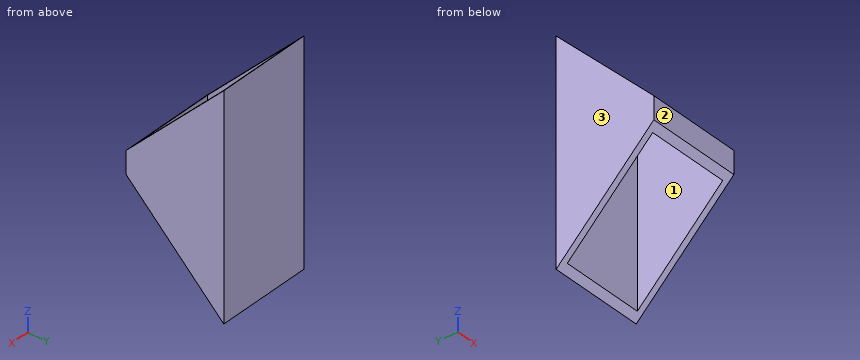
```python
from build123d import *

# Parameters (mm, degrees)
CROQUIS2_W              = 76.2
CROQUIS2_H              = 76.2
CROQUIS2_W_2            = 66.675
CROQUIS2_H_2            = 66.675
SALIENTE_EXTRUIR1_DEPTH = 170
CORTAR_EXTRUIR1_REACH   = 203.278


with BuildPart() as part:
    # Croquis2 → Saliente-Extruir1 (new body)
    with BuildSketch(Plane.XY):
        with Locations((38.1, -38.1)):
            Rectangle(CROQUIS2_W, CROQUIS2_H)
        with Locations((38.1, -38.1)):
            Rectangle(CROQUIS2_W_2, CROQUIS2_H_2, mode=Mode.SUBTRACT)
    extrude(amount=-SALIENTE_EXTRUIR1_DEPTH)

    # Cortar-Extruir1: up to this face of the body (flat: up to its plane)
    cortar_extruir1_end = Plane(part.part.faces().sort_by_distance((0, -38.1, -85))[0])
    # Croquis3 → Cortar-Extruir1 (cut, up to the picked face)
    with BuildSketch(Plane(origin=(76.2, 0, 0), x_dir=(0, 0, -1), z_dir=(1, 0, 0)), mode=Mode.PRIVATE) as cortar_extruir1_sk1:
        Polygon((0, 0), (76.2, -76.2), (0, -76.2), align=None)
    cortar_extruir1_tool1 = split(extrude(cortar_extruir1_sk1.sketch, amount=-CORTAR_EXTRUIR1_REACH, mode=Mode.PRIVATE), bisect_by=cortar_extruir1_end, keep=Keep.BOTH, mode=Mode.PRIVATE)
    # Croquis3 → Cortar-Extruir1 (cut, up to the picked face)
    with BuildSketch(Plane(origin=(76.2, 0, 0), x_dir=(0, 0, -1), z_dir=(1, 0, 0)), mode=Mode.PRIVATE) as cortar_extruir1_sk2:
        Polygon((170, 0), (93.8, -76.2), (170, -76.2), align=None)
    cortar_extruir1_tool2 = split(extrude(cortar_extruir1_sk2.sketch, amount=-CORTAR_EXTRUIR1_REACH, mode=Mode.PRIVATE), bisect_by=cortar_extruir1_end, keep=Keep.BOTH, mode=Mode.PRIVATE)
    add(cortar_extruir1_tool1.solids().sort_by(Axis((76.2, -50.8, -25.4), (-1, 0, 0)))[0], mode=Mode.SUBTRACT)
    add(cortar_extruir1_tool2.solids().sort_by(Axis((76.2, -50.8, -144.6), (-1, 0, 0)))[0], mode=Mode.SUBTRACT)


solid = part.part
```
Verification items for the finished model (mm, model axes). Face numbers are marked on the shaded views. Coordinates: 2 decimals unless noted, no trailing zeros. Loops run counter-clockwise (first coordinate to the right, second up) from the corner with the lowest first, then second, coordinate; pieces in that order, holes last. Notation, with made-up numbers: (71.5, 47) -> (124.5, 47) arc R17 ccw to (124.5, 65) -> close; hole circle Ø7 at (28, 39). An arc over 180 degrees is marked (long way). Answer in a Markdown table with one row per item. Add a question column.
1. Section check A-A, the plane y = -56. Enter the section's corners in (x, z), then the cut area to 3 significant figures.
2. Material ranges on probe 1 along X at (y, z) = (-40.5, -114.5); probe 2 along Y at (x, z) = (52, -51); probe 3 along Z at (x, y) = (71.5, -47), recorded low to high. Write a range as [from, to].
3. Depth check by flat-ended pin: P1, Ø12, axis at x = 58, z = -19.5, coming from the +Y side; P2, Ø12, axis at x = 44.5, z = -35, coming from the -Y side. Enter the tip coordinate at first touch or a pass-through.
4. Draft check along Y on the marked faces 1, 2 and 3. Enter one of: +Y half, -Y half, draft (parallel to the pull), parting line (faces both ways), or undercut.
5. Section check C-C, the plane z = -45. Enter the section's corners in (x, y), then the cut area to 3 significant figures.
6. Section check D-D, the plane z = -128.5. Enter the section's corners in (x, y).
7. Section check B-B, the plane x = 22. Enter the section's corners in (y, z), then the cut area to 3 significant figures.
Derived:
| question | item | result |
|---|---|---|
| 1 | outline | (0, -114) -> (4.76, -114) -> (4.76, -56) -> (0, -56) -> close; (71.44, -114) -> (76.2, -114) -> (76.2, -56) -> (71.44, -56) -> close |
| 1 | area | 552 mm² |
| 2 | probe 1 | x = [0, 4.76], [71.44, 76.2] |
| 2 | probe 2 | y = [-4.76, 0] |
| 2 | probe 3 | z = [-123, -47] |
| 3 | P1 | stops at y = 0 |
| 3 | P2 | stops at y = -4.76 |
| 4 | face 1 | undercut |
| 4 | face 2 | -Y half |
| 4 | face 3 | draft |
| 5 | outline | (0, -45) -> (4.76, -45) -> (4.76, -4.76) -> (71.44, -4.76) -> (71.44, -45) -> (76.2, -45) -> (76.2, 0) -> (0, 0) -> close |
| 5 | area | 746 mm² |
| 6 | outline | (0, -41.5) -> (4.76, -41.5) -> (4.76, -4.76) -> (71.44, -4.76) -> (71.44, -41.5) -> (76.2, -41.5) -> (76.2, 0) -> (0, 0) -> close |
| 7 | outline | (-76.2, -93.8) -> (-71.44, -98.56) -> (-71.44, -71.44) -> (-76.2, -76.2) -> close; (-4.76, -165.24) -> (0, -170) -> (0, 0) -> (-4.76, -4.76) -> close |
| 7 | area | 893 mm² |
